from build123d import *

# Parameters (mm, degrees)
REVOLVE1_ANGLE                                      = 110
CSK_FOR_M3_COUNTERSUNK_FLAT_HEAD_SCREW1_D           = 3.4
CSK_FOR_M3_COUNTERSUNK_FLAT_HEAD_SCREW1_CSINK_D     = 6.3
CSK_FOR_M3_COUNTERSUNK_FLAT_HEAD_SCREW1_CSINK_ANGLE = 90


with BuildPart() as part:
    # Sketch1 → Revolve1 (revolve)
    with BuildSketch(Plane.XY):
        Polygon((-29, 0), (-29, 8), (-40, 8), (-39.896417966, 0.000670605), align=None)
    revolve(axis=Axis((0, 0, 0), (0, 1, 0)), revolution_arc=REVOLVE1_ANGLE)

    # CSK for M3 Countersunk Flat Head Screw1 (through all)
    with Locations(Plane(origin=(-16.693228701, 3.799474552, 23.713627212), x_dir=(-0.817711283, 0, -0.575628576), z_dir=(0.575628576, 0, -0.817711283))):
        with Locations((0, 0)):
            CounterSinkHole(CSK_FOR_M3_COUNTERSUNK_FLAT_HEAD_SCREW1_D / 2, CSK_FOR_M3_COUNTERSUNK_FLAT_HEAD_SCREW1_CSINK_D / 2, counter_sink_angle=CSK_FOR_M3_COUNTERSUNK_FLAT_HEAD_SCREW1_CSINK_ANGLE)


solid = part.part
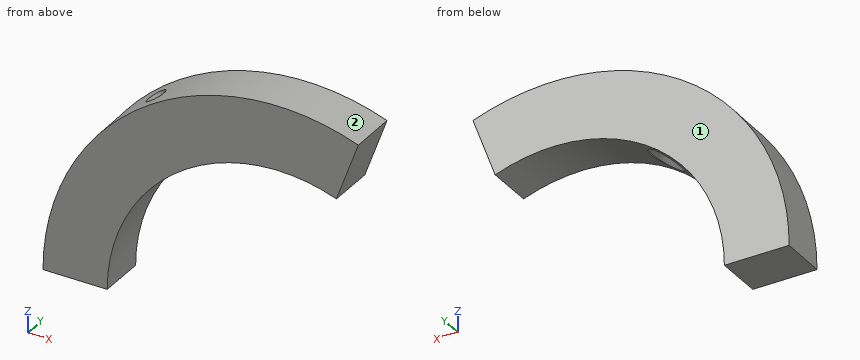
Geometry: final body of the model. Coordinates: model frame, mm. Face numbers are marked on the shaded views. A direction names the side the tool comes from. Give positions to 0.01 mm unless a question says otherwise; leave off trailing zeros. One line per question, with ' | ' between items. Start each with the question number.
(1) Contact query for flat-ended pins moving along their axis: pin 1 (3 mm diameter, centred on x = -11.5, y = 4.5, fed in from -Z); pin 2 (2 mm diameter, centred on y = 1.5, z = 13.5, fed in from -X). Output: stop coordinate, or through.
(2) Ray query, line 1 (X direction, y = 0.5, z = 16); line 2 (Z direction, x = -9.5, y = 2); line 3 (X direction, y = 5.5, z = 23.5). Return the intervals inside material, ascending. Write a range as from..to.
(3) Reachability of the marked faces 1 and 2 from +Z, -Z, +X, -X, +Y, -Y: full face, straight path, thin tool, end or side. Return the list, or none.
The answers:
1) pin 1: z = 25.92 | pin 2: x = -37.91
2) line 1: -36.55..-24.19 | line 2: 27.4..38.78 | line 3: -32.33..-18.46
3) face 1: +Z, -Z, +X, -X, +Y | face 2: +Z, -Y
